Input: part model. Units: mm. Frame: model coordinates. A direction names the side the tool comes from. Round coordinates to 2 decimals unless told otherwise and drop trailing zeros. Loops run counter-clockwise (first coordinate to the right, second up) from the corner with the lowest first, then second, coordinate; pieces in that order, holes last. Notation, with made-up numbers: (69.25, 86.25) -> (98.25, 86.25) arc R21 cw to (98.25, 114.25) -> close; hole circle Ø7 at (25.25, -23.75). An arc over 180 degrees is marked (long way). Answer in a Markdown table with one row per item. Add a question column.
Q1. Section A-A, the plane x = 53. Output: boundary loops of the cut face in (y, z) (3 decimals).
Q2. Section D-D, the plane z = 23. Output: boundary loops of the cut face in (x, y) (3 decimals).
Q3. Reachability of faces 1 (the face through (59, 44.45, 1)), 2 (the face through (46, 24, 16.375)), 3 (the face through (61.81, 24, 0)), 4 (the face through (45, 24, 13.2)) from +Z, -Z, +X, -X, +Y, -Y: full face, straight path, thin tool, end or side. Return the list, or none.
Q4. Pin query (flat end, axial travel): pin 1 (13.5 mm diameter, centred on x = 51, y = 33.5, fed in from -Z) (3 decimals); pin 2 (5 mm diameter, centred on x = 6, z = -35.5, fed in from +Y) (3 decimals); pin 3 (21 mm diameter, centred on y = 26.5, z = 5.5, fed in from -X). Return the tip coordinate at first contact, or that it passes through.
Q5. Section B-B, the plane y = 23. Output: boundary loops of the cut face in (x, z) (3 decimals).
Q6. Mould query, pull axis Z, two halves, no side actions, for faces 5 (the face through (47, 24, -16.375)), 6 (the face through (45, 24, -13.2)), 7 (the face through (-1, 0, -1)). Classes: pulls with the +Z half, pulls with the -Z half, needs draft (parallel to the pull), parting line crosses it, or undercut.
Q7. Section C-C, the plane z = 3. Output: boundary loops of the cut face in (x, y) (3 decimals), and give its area (3 significant figures).
Q8. Ray query, L1, parallel to Z at x = 41, y = 36.5 (3 decimals); L2, parallel to Y at x = -22, z = 36.5 (3 decimals); L3, parallel to X at y = 13.5, z = 1.5. Return the intervals inside material, ascending. Write a range as from..to.
```python
from build123d import *

# Parameters (mm, degrees)
SKETCH1_W           = 152.4
SKETCH1_H           = 152.4
BOSS_EXTRUDE1_DEPTH = 3.175
BOSS_EXTRUDE2_DEPTH = 41.275


with BuildPart() as part:
    # Sketch1 → Boss-Extrude1 (new body)
    with BuildSketch(Plane(origin=(0, 0, 0), x_dir=(1, 0, 0), z_dir=(0, 1, 0))):
        Rectangle(SKETCH1_W, SKETCH1_H)
    extrude(amount=BOSS_EXTRUDE1_DEPTH)

    # Sketch2 → Boss-Extrude2 (add)
    with BuildSketch(Plane(origin=(0, 3.175, 0), x_dir=(1, 0, 0), z_dir=(0, 1, 0))):
        Polygon((58.635483549, 13.2), (58.635483549, 0), (61.810483549, 0), (61.810483549, 16.375), (31.535483549, 16.375), (31.535483549, 13.266442451), (31.535483549, 13.2), align=None)
        Polygon((61.810483549, 0), (58.635483549, 0), (58.635483549, -13.2), (31.535483549, -13.2), (31.535483549, -16.375), (61.810483549, -16.375), align=None)
    extrude(amount=BOSS_EXTRUDE2_DEPTH)


solid = part.part
```
Answer block:
| question | item | result |
|---|---|---|
| 1 | outline | (0, -76.2) -> (3.175, -76.2) -> (3.175, -16.375) -> (44.45, -16.375) -> (44.45, -13.2) -> (3.175, -13.2) -> (3.175, 13.2) -> (44.45, 13.2) -> (44.45, 16.375) -> (3.175, 16.375) -> (3.175, 76.2) -> (0, 76.2) -> close |
| 2 | outline | (-76.2, 0) -> (76.2, 0) -> (76.2, 3.175) -> (-76.2, 3.175) -> close |
| 3 | face 1 | +Z, -Z, +X, -X, +Y |
| 3 | face 2 | +Z, +X, -X, +Y |
| 3 | face 3 | +Z, -Z, +X, +Y |
| 3 | face 4 | -X, +Y |
| 4 | pin 1 | z = -16.375 |
| 4 | pin 2 | y = 3.175 |
| 4 | pin 3 | x = 31.54 |
| 5 | outline | (31.535, -16.375) -> (61.81, -16.375) -> (61.81, 16.375) -> (31.535, 16.375) -> (31.535, 13.2) -> (58.635, 13.2) -> (58.635, -13.2) -> (31.535, -13.2) -> close |
| 6 | face 5 | pulls with the -Z half |
| 6 | face 6 | undercut |
| 6 | face 7 | needs draft |
| 7 | outline | (-76.2, 0) -> (76.2, 0) -> (76.2, 3.175) -> (61.81, 3.175) -> (61.81, 44.45) -> (58.635, 44.45) -> (58.635, 3.175) -> (-76.2, 3.175) -> close |
| 7 | area | 615 mm^2 |
| 8 | L1 | -16.375..-13.2, 13.2..16.375 |
| 8 | L2 | 0..3.175 |
| 8 | L3 | 58.64..61.81 |
